Can you work these out from the model? Positions are in its coordinate system, mm. A direction names the side the tool comes from. Give positions to 0.01 mm unless a question says otherwise; leave off trailing zeros. Loops run counter-clockwise (first coordinate to the right, second up) from the corner with the lowest first, then second, coordinate; pieces in that order, holes last. Notation, with made-up numbers: M -26,71.25 L 17,71.25 A18 cw 17,84.25 Z; hole C -20.75,64.5 d8. An arc over 180 degrees is marked long. Use CSV: the item, a comma, the result in double quotes.
from build123d import *

# Parameters (mm, degrees)
BOSS_EXTRUDE2_DEPTH = 30
SKETCH2_W           = 10
SKETCH2_H           = 14
SKETCH2_R           = 2.25
SKETCH2_R_2         = 2.75
BOSS_EXTRUDE3_DEPTH = 4
SKETCH6_R           = 4
CUT_EXTRUDE1_DEPTH  = 2
BOSS_EXTRUDE4_DEPTH = 50
SKETCH8_W           = 10
SKETCH8_H           = 14
SKETCH8_R           = 2.75
BOSS_EXTRUDE5_DEPTH = 4


with BuildPart() as part:
    # Sketch1 → Boss-Extrude2 (new, symmetric)
    with BuildSketch(Plane(origin=(0, 0, 0), x_dir=(0, 0, -1), z_dir=(1, 0, 0))):
        with BuildLine():
            Line((-13.919410907, 1.5), (-9.886859967, 1.5))
            ThreePointArc((-9.886859967, 1.5), (0, 10), (9.886859967, 1.5))
            Line((9.886859967, 1.5), (13.919410907, 1.5))
            ThreePointArc((13.919410907, 1.5), (0, 14), (-13.919410907, 1.5))
        make_face()
    extrude(amount=BOSS_EXTRUDE2_DEPTH, both=True)

    # Sketch2 → Boss-Extrude3 (add)
    # profile 1 of 6: a face of its own
    with BuildSketch(Plane.XZ.offset(-1.5)):
        with Locations((-25, -16.886859967)):
            Rectangle(SKETCH2_W, SKETCH2_H)
        with Locations(Location((-25, -18.903135437, 0), (0, 0, 270))):
            Circle(SKETCH2_R, mode=Mode.SUBTRACT)
    # profile 2 of 6: a face of its own
    with BuildSketch(Plane.XZ.offset(-1.5)):
        with Locations((25, -16.886859967)):
            Rectangle(SKETCH2_W, SKETCH2_H)
        with Locations(Location((25, -18.903135437, 0), (0, 0, 270))):
            Circle(SKETCH2_R, mode=Mode.SUBTRACT)
    # profile 3 of 6: a face of its own
    with BuildSketch(Plane.XZ.offset(-1.5)):
        with Locations((-25, 16.886859967)):
            Rectangle(SKETCH2_W, SKETCH2_H)
        with Locations(Location((-25, 18.903135437, 0), (0, 0, 270))):
            Circle(SKETCH2_R, mode=Mode.SUBTRACT)
    # profile 4 of 6: a face of its own
    with BuildSketch(Plane.XZ.offset(-1.5)):
        with Locations((25, 16.886859967)):
            Rectangle(SKETCH2_W, SKETCH2_H)
        with Locations(Location((25, 18.903135437, 0), (0, 0, 270))):
            Circle(SKETCH2_R, mode=Mode.SUBTRACT)
    # profile 5 of 6: a face of its own
    with BuildSketch(Plane.XZ.offset(-1.5)):
        with Locations((0, 16.886859967)):
            Rectangle(SKETCH2_W, SKETCH2_H)
        with Locations(Location((0, 18.903135437, 0), (0, 0, 270))):
            Circle(SKETCH2_R_2, mode=Mode.SUBTRACT)
    # profile 6 of 6: a face of its own
    with BuildSketch(Plane.XZ.offset(-1.5)):
        with Locations((0, -16.886859967)):
            Rectangle(SKETCH2_W, SKETCH2_H)
        with Locations(Location((0, -18.903135437, 0), (0, 0, 90))):
            Circle(SKETCH2_R_2, mode=Mode.SUBTRACT)
    extrude(amount=-BOSS_EXTRUDE3_DEPTH)

    # Sketch6 → Cut-Extrude1 (cut)
    with BuildSketch(Plane.XZ.offset(-1.5)):
        with Locations(Location((-25, 18.903135437, 0), (0, 0, 270))):
            Circle(SKETCH6_R)
        with Locations(Location((25, -18.903135437, 0), (0, 0, 270))):
            Circle(SKETCH6_R)
        with Locations(Location((-25, -18.903135437, 0), (0, 0, 270))):
            Circle(SKETCH6_R)
        with Locations(Location((25, 18.903135437, 0), (0, 0, 270))):
            Circle(SKETCH6_R)
    extrude(amount=-CUT_EXTRUDE1_DEPTH, mode=Mode.SUBTRACT)

    # Sketch7 → Boss-Extrude4 (add)
    with BuildSketch(Plane.ZY.offset(30)):
        with BuildLine():
            Line((-14.924811557, 1.5), (-10.897247359, 1.5))
            ThreePointArc((-10.897247359, 1.5), (0, 11), (10.897247359, 1.5))
            Line((10.897247359, 1.5), (14.924811557, 1.5))
            ThreePointArc((14.924811557, 1.5), (0, 15), (-14.924811557, 1.5))
        make_face()
    boss_extrude4 = extrude(amount=BOSS_EXTRUDE4_DEPTH)

    # Sketch8 → Boss-Extrude5 (add)
    # profile 1 of 4: a face of its own
    with BuildSketch(Plane.XZ.offset(-1.5)):
        with Locations((-75, 17.897247359)):
            Rectangle(SKETCH8_W, SKETCH8_H)
        with Locations(Location((-75, 19.911029458, 0), (0, 0, 270))):
            Circle(SKETCH8_R, mode=Mode.SUBTRACT)
    # profile 2 of 4: a face of its own
    with BuildSketch(Plane.XZ.offset(-1.5)):
        with Locations((-35, 17.897247359)):
            Rectangle(SKETCH8_W, SKETCH8_H)
        with Locations(Location((-35, 19.911029458, 0), (0, 0, 90))):
            Circle(SKETCH8_R, mode=Mode.SUBTRACT)
    # profile 3 of 4: a face of its own
    with BuildSketch(Plane.XZ.offset(-1.5)):
        with Locations((-75, -17.897247359)):
            Rectangle(SKETCH8_W, SKETCH8_H)
        with Locations(Location((-75, -19.911029458, 0), (0, 0, 90))):
            Circle(SKETCH8_R, mode=Mode.SUBTRACT)
    # profile 4 of 4: a face of its own
    with BuildSketch(Plane.XZ.offset(-1.5)):
        with Locations((-35, -17.897247359)):
            Rectangle(SKETCH8_W, SKETCH8_H)
        with Locations(Location((-35, -19.911029458, 0), (0, 0, 270))):
            Circle(SKETCH8_R, mode=Mode.SUBTRACT)
    boss_extrude5 = extrude(amount=-BOSS_EXTRUDE5_DEPTH)

    # Mirror1: Boss-Extrude4, Boss-Extrude5 across plane
    add(boss_extrude4.mirror(Plane(origin=(0, 0, 0), x_dir=(0, 0, 1), z_dir=(1, 0, 0))))
    add(boss_extrude5.mirror(Plane(origin=(0, 0, 0), x_dir=(0, 0, 1), z_dir=(1, 0, 0))))


solid = part.part
Q1. I want a section at A-A, the plane x = 0. Please give me the cut outline in (y, z).
Model answer:
outline,"M 1.5,-23.89 L 5.5,-23.89 L 5.5,-21.65 L 1.5,-21.65 Z; M 1.5,-16.15 L 5.5,-16.15 L 5.5,-12.87 A14 ccw 5.5,12.87 L 5.5,16.15 L 1.5,16.15 L 1.5,9.89 A10 cw 1.5,-9.89 Z; M 1.5,21.65 L 5.5,21.65 L 5.5,23.89 L 1.5,23.89 Z"
Q2. For faces 4 (the cylindrical face through (55, 15, 0)), 5 (the flat face through (-19, 1.5, 12)), 6 (the flat face through (-25, 3, 23.887)), 7 (the flat face through (-27, 3.5, -21)), which set-ups out of +Z, -Z, +X, -X, +Y, -Y let a thin tool reach every point of the face, with its end or its side?
Model answer:
face 4,"+Y"
face 5,"+Z, -Z, +X, -X, -Y"
face 6,"+Z, +Y, -Y"
face 7,"-Y"
Q3. Please list where these lines run through material, in increasing order: L1, parallel to X at y = 11.75, z = -8.5; L2, parallel to Z at x = -25.5, y = 4.5; L3, parallel to Z at x = 5.5, y = 2.75. Write a range as from..to.
Model answer:
L1,"-80..-30, 30..80"
L2,"-23.89..-21.1, -16.71..-8.93, 8.93..16.71, 21.1..23.89"
L3,"-13.73..-9.61, 9.61..13.73"
Q4. I want a section at B-B, the plane x = -35. Please give me the cut outline in (y, z).
Model answer:
outline,"M 1.5,-24.9 L 5.5,-24.9 L 5.5,-22.66 L 1.5,-22.66 Z; M 1.5,-17.16 L 5.5,-17.16 L 5.5,-13.96 A15 ccw 5.5,13.96 L 5.5,17.16 L 1.5,17.16 L 1.5,10.9 A11 cw 1.5,-10.9 Z; M 1.5,22.66 L 5.5,22.66 L 5.5,24.9 L 1.5,24.9 Z"
Q5. If we mould it in two halves opening along X, with no side actions, what happens to faces 1 (the flat face through (25, 3, -23.887)), 2 (the cylindrical face through (-26.37, 4.49, -17.12)), 3 (the flat face through (-75, 5.5, 17))? For each: released by +X, released by -X, zero draft, split by the parting line, or undercut.
Model answer:
face 1,"undercut"
face 2,"undercut"
face 3,"zero draft"
Q6. I'm going to push flat-ended pins straight in: P1, Ø4.5, axis at x = 0, z = -18.9, coming from the -Y side (3 decimals); P2, Ø10, axis at x = -13.5, z = 9, coming from the +Y side; P3, Ø3, axis at x = 75.5, z = -18.5, coming from the +Y side; P4, Ø2.5, axis at x = 25, z = 20, coming from the -Y side. Where does each tip first touch, or does it pass through?
Model answer:
P1,"through"
P2,"y = 13.42"
P3,"y = 5.5"
P4,"y = 3.5"
Q7. I want a section at C-C, the plane z = 5. Please give me the cut outline in (x, y).
Model answer:
outline,"M -80,9.8 L -30,9.8 L -30,8.66 L 30,8.66 L 30,9.8 L 80,9.8 L 80,14.14 L 30,14.14 L 30,13.08 L -30,13.08 L -30,14.14 L -80,14.14 Z"
